Geometry check sheet. Reference: drawing and pictorial views, mm from the part's lowest x, y, z. A direction names the side the tool comes from. Round coordinates to 2 decimals unless told otherwise and drop trailing zeros. Write each loop counter-clockwise with the first axis right and the second up, starting at its lowest first coordinate (ties: lowest second). Pieces come first, ordered by that corner, then holes. Notation, with made-up numbers: (67.25, 13.5) -> (95.25, 13.5) arc R25 cw to (95.25, 31.5) -> close; hole circle Ø6 at (64.5, 10.25). An arc over 180 degrees is marked (long way). Answer as a JSON object with one key per item and string values. Group by question number.
(1) Draft check along Y on the marked faces 4, 5 and 6. Enter one of: released by +Y, released by -Y, zero draft, split by the parting line, or undercut.
(2) Sectioned sample at D-D on y = 48. Record the cut outline in (x, z), and give its area (3 significant figures).
(3) Scan lines: L1, parallel to Y at x = 34, z = 5.5; L2, parallel to X at y = 38, z = 3; L3, parallel to Y at x = 2.5, z = 22.5. Record each from-to range of solid material in increasing order. Write a range as from..to.
(4) Sectioned sample at A-A on x = 36.5. Record the cut outline in (y, z).
(5) Set-up check for the marked faces 1, 2 and 3: record each of +Z, -Z, +X, -X, +Y, -Y from which the full face is reachable in a straight line by a thin tool's end or side.
(6) Gauge pin test, flat ends, axial feed: pin 1 Ø5 at (y, z) = (38.5, 37) entering from +X; pin 2 Ø10 at (y, z) = (7.5, 20.5) entering from -X; pin 3 Ø3 at (x, z) = (7.5, 17.5) entering from -Y. Record the tip position at first contact, or that the pin passes through.
(7) Sectioned sample at B-B on z = 29. Record the cut outline in (x, y).
(8) Sectioned sample at C-C on x = 45. Record the cut outline in (y, z).
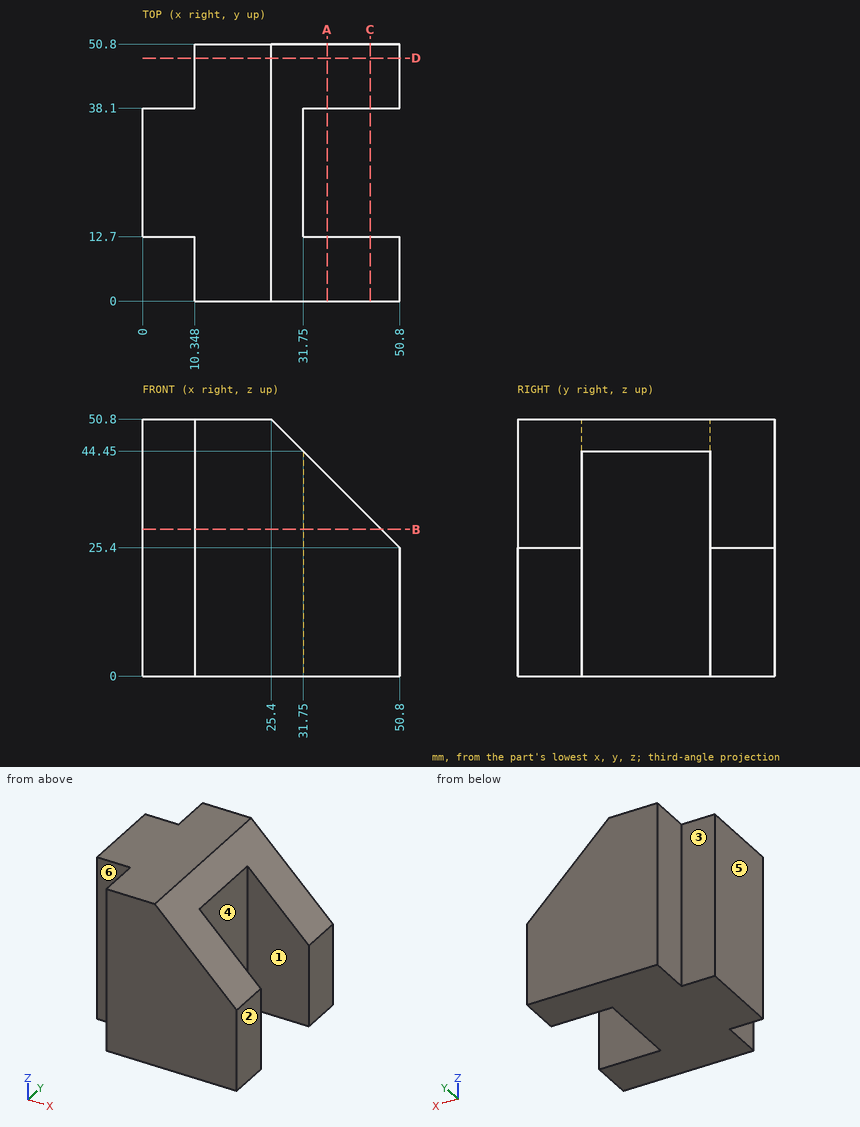
Computed values:
{
 "1": {"face 4": "undercut", "face 5": "zero draft", "face 6": "released by -Y"},
 "2": {"outline": "(10.35, 0) -> (50.8, 0) -> (50.8, 25.4) -> (25.4, 50.8) -> (10.35, 50.8) -> close", "area": "1,730 mm2"},
 "3": {"L1": "0..12.7, 38.1..50.8", "L2": "0..31.75", "L3": "12.7..38.1"},
 "4": {"outline": "(0, 0) -> (12.7, 0) -> (12.7, 39.7) -> (0, 39.7) -> close; (38.1, 0) -> (50.8, 0) -> (50.8, 39.7) -> (38.1, 39.7) -> close"},
 "5": {"face 1": "+Z, -Z, +X", "face 2": "+Z, -Z, +X, +Y, -Y", "face 3": "+Z, -Z, -X, +Y"},
 "6": {"pin 1": "x = 41.7", "pin 2": "x = 10.35", "pin 3": "y = 12.7"},
 "7": {"outline": "(0, 12.7) -> (10.35, 12.7) -> (10.35, 0) -> (47.2, 0) -> (47.2, 12.7) -> (31.75, 12.7) -> (31.75, 38.1) -> (47.2, 38.1) -> (47.2, 50.8) -> (10.35, 50.8) -> (10.35, 38.1) -> (0, 38.1) -> close"},
 "8": {"outline": "(0, 0) -> (12.7, 0) -> (12.7, 31.2) -> (0, 31.2) -> close; (38.1, 0) -> (50.8, 0) -> (50.8, 31.2) -> (38.1, 31.2) -> close"}
}
